```python
from build123d import *

# Parameters (mm, degrees)
F0_W     = 89
F0_H     = 18
F1_DEPTH = 18
F2_R     = 5


with BuildPart() as f1:
    # F0 (on Top) → F1 (new body)
    with BuildSketch(Plane.XY):
        with Locations((44.5, 9)):
            Rectangle(F0_W, F0_H)
    extrude(amount=F1_DEPTH)

    # F2
    f2_edges = [f1.edges().sort_by_distance(p)[0] for p in [
        (0, 0, 9),
        (89, 0, 9),
        (89, 18, 9),
        (0, 18, 9),
        (0, 9, 18),
        (89, 9, 18),
    ]]
    fillet(f2_edges, radius=F2_R)


solid = f1.part
```
For this review, take the finished solid that the model builds, in its own axes (mm). Round coordinates to 2 decimals unless told otherwise and drop trailing zeros. Loops run counter-clockwise (first coordinate to the right, second up) from the corner with the lowest first, then second, coordinate; pieces in that order, holes last.
(1) Clearance check with flat-ended pins moving along their axes: P1, Ø2, axis at y = 2, z = 14, coming from the +X side; P2, Ø5, axis at y = 3, z = 15, coming from the -X side. State where each tip first meets the part, or that it passes through.
Returned:
P1: stops at x = 88.58
P2: stops at x = 0.01
(2) We need section B-B (y = 17). Give the boundary of the cut face in (x, z), plus the area to 3 significant figures.
Returned:
outline: (2, 0) - (87, 0) - (87, 17) arc R5 ccw to (84, 18) - (5, 18) arc R5 ccw to (2, 17) - close
area: 1,530 mm2
(3) We need section A-A (z = 16). Give the boundary of the cut face in (x, y).
Returned:
outline: (1, 2) arc R5 ccw to (5, 0) - (84, 0) arc R5 ccw to (88, 2) - (88, 16) arc R5 ccw to (84, 18) - (5, 18) arc R5 ccw to (1, 16) - close
(4) Wall thickness on line 1 along X through (y, z) = (4.5, 10); line 2 along X through (y, z) = (15.75, 6): over which ranges is each line inside the solid? List them lowest first.
Returned:
line 1: x = 0.03 to 88.97
line 2: x = 0.82 to 88.18
